Autodesk Inventor part; units mm, degrees
ref_plane "Work Plane1" through (0, -6.3, 0) normal (0, 0, 1) x (1, 0, 0)
ref_plane "YZ Plane" through (0, 0, 0) normal (1, 0, 0) x (0, 1, 0)
ref_plane "XZ Plane" through (0, 0, 0) normal (0, 1, 0) x (-1, 0, 0)
sketch "Sketch2" plane through (0, 0, 0) normal (1, 0, 0) x (0, 1, 0)
  line L0 (-6.3, 8.85) -> (6.3, 8.85)
  line L1 (6.3, 8.85) -> (6.3, -8.85)
  line L2 (6.3, -8.85) -> (-6.3, -8.85)
  line L3 (-6.3, -8.85) -> (-6.3, 8.85)
  line L4 (-6.3, 8.85) -> (6.3, -8.85) construction
  line L5 (6.3, 8.85) -> (-6.3, -8.85) construction
  point P0 (0, 0)
  dimension "d0" = 17.7
  dimension "d1" = 12.6
extrude "Extrusion1" add sketch "Sketch2" along normal blind 11.5
fillet "Fillet1" radius 1 3 edges at (5.75, 6.3, 8.85) (5.75, 6.3, -8.85) (0, 6.3, 0)
ref_plane "Work Plane1" through (0, -6.3, 0) normal (0, 0, 1) x (1, 0, 0)
sketch "Sketch3" plane through (11.5, 0, 0) normal (1, 0, 0) x (0, 0, -1)
  circle A0 centre (-4, 0) radius 1.25
  point P0 (0, 0)
  dimension "d5" = 2.5
  dimension "d6" = 4
hole "Hole1" at (11.5, 0, 4) direction (-1, 0, 0) diameter 2.5 depth 1
mirror "Mirror1" about plane through (0, -6.3, 0) normal (0, 0, 1) of "Hole1"
properties part number "IR sensor" material "ABS Plastic"
For this review, take the finished solid that the model builds, in its own axes (mm). A direction names the side the tool comes from. Give positions to 0.01 mm unless a question says otherwise; leave off trailing zeros. Loops run counter-clockwise (first coordinate to the right, second up) from the corner with the lowest first, then second, coordinate; pieces in that order, holes last.
Item 1: Tool access review of faces 5 (the cylindrical face through (5.83, 6.015, 8.549)), 6 (the cylindrical face through (10.99, 0.05, -5.25)): name each direction out of +Z, -Z, +X, -X, +Y, -Y from which nothing blocks a thin tool from reaching the whole face with its end or side.
Item 2: For line 1 along Z through (x, y) = (11.15, 0); line 2 along Y through (x, z) = (10.95, -4); line 3 along X through (y, z) = (-1, 4.5), list the stretches that pass through material, from the lowest coordinate up.
Item 3: Draft analysis for pull direction Z (two halves, no side actions). For faces 1 (the flat face through (11.5, 0, 0)), 2 (the flat face through (10.5, 0, 4)), 3 (the flat face through (6, 0, -8.85)), 4 (the flat face through (6, -1, 8.85)), state which applies: +Z half, -Z half, draft (parallel to the pull), parting line (faces both ways), or undercut.
Item 4: Take a section at B-B, the plane y = 0. State the section outline as (x, z) points.
Item 5: Take a section at A-A, the plane z = 4. State the section outline as (x, y) points, and give its area (3 significant figures).
Item 6: Insertion check: pin 1 (0.8 mm diameter, centred on y = 0.5, z = -3.5, fed in from +X). The pin has a flat end and moves straight along its axis. Give the tip position at first contact, or say it passes through.
Calculated:
1. face 5: +Z, +X, -X, +Y
1. face 6: +X
2. line 1: z = -8.85 to -5.25, -2.75 to 2.75, 5.25 to 8.85
2. line 2: y = -6.3 to -1.25, 1.25 to 6.3
2. line 3: x = 0 to 10.5
3. face 1: draft
3. face 2: undercut
3. face 3: -Z half
3. face 4: +Z half
4. outline: (0, -8.85) - (11.5, -8.85) - (11.5, -5.25) - (10.5, -5.25) - (10.5, -2.75) - (11.5, -2.75) - (11.5, 2.75) - (10.5, 2.75) - (10.5, 5.25) - (11.5, 5.25) - (11.5, 8.85) - (0, 8.85) - close
5. outline: (0, -6.3) - (11.5, -6.3) - (11.5, -1.25) - (10.5, -1.25) - (10.5, 1.25) - (11.5, 1.25) - (11.5, 6.3) - (1, 6.3) arc R1 ccw to (0, 5.3) - close
5. area: 142 mm2
6. pin 1: stops at x = 10.5
